The model under review builds one solid part; all positions refer to its coordinate system, in mm. A direction names the side the tool comes from. Coordinates: 2 decimals unless noted, no trailing zeros. Order: outer loops, then holes, each group sorted by start corner. A loop starts at its lowest first (then second) coordinate and runs counter-clockwise, first axis right, second up. Notation, with made-up numbers: (76, 79.5) - (120, 79.5) arc R18 cw to (120, 103.5) - close; hole circle Ø2 at (-24, 71.5). An arc over 180 degrees is marked (long way). Answer in a Markdown table with one row per item.
```python
from build123d import *

# Parameters (mm, degrees)
F0_W     = 17
F0_H     = 17
F1_DEPTH = 1
F2_W     = 14
F2_H     = 14
F3_DEPTH = 1
F4_R     = 0.49999


# Not quite as in the source:
# - a fillet or chamfer is up to 0.001 mm smaller than in the source, because OpenCascade refuses the exact size


with BuildPart() as f1:
    # F0 (on Top) → F1 (new body)
    with BuildSketch(Plane.XY):
        with Locations((-37.4565784931, 18.6608627687)):
            Rectangle(F0_W, F0_H)
    extrude(amount=F1_DEPTH)

    # F2 (on face) → F3 (join)
    with BuildSketch(Plane.XY.offset(1)):
        with Locations((-37.4565784931, 18.6608627687)):
            Rectangle(F2_W, F2_H)
    extrude(amount=F3_DEPTH)

    # F4 (radius 0.5 in the source; OpenCascade refuses exactly that, so slightly less here)
    f4_edges = [f1.edges().sort_by_distance(p)[0] for p in [
        (-37.456578, 25.660863, 2),
        (-44.456578, 18.660863, 2),
        (-44.456578, 18.660863, 1),
        (-37.456578, 25.660863, 1),
        (-37.456578, 11.660863, 2),
        (-37.456578, 10.160863, 1),
        (-45.956578, 18.660863, 1),
        (-45.956578, 18.660863, 0),
        (-45.956578, 27.160863, 0.5),
        (-37.456578, 27.160863, 1),
        (-37.456578, 27.160863, 0),
        (-30.456578, 18.660863, 1),
        (-30.456578, 18.660863, 2),
        (-30.456578, 25.660863, 1.5),
        (-28.956578, 18.660863, 1),
        (-28.956578, 18.660863, 0),
        (-28.956578, 27.160863, 0.5),
        (-28.956578, 10.160863, 0.5),
        (-45.956578, 10.160863, 0.5),
        (-37.456578, 10.160863, 0),
        (-37.456578, 11.660863, 1),
        (-44.456578, 11.660863, 1.5),
        (-30.456578, 11.660863, 1.5),
    ]]
    fillet(f4_edges, radius=F4_R)


solid = f1.part
```
Item 1: We need section C-C, the plane z = 0.75. Write out the cut boundary in (x, y).
Check values:
| item | result |
|---|---|
| outline | (-45.89, 10.66) arc R0.43 ccw to (-45.46, 10.23) - (-29.46, 10.23) arc R0.43 ccw to (-29.02, 10.66) - (-29.02, 26.66) arc R0.43 ccw to (-29.46, 27.09) - (-45.46, 27.09) arc R0.43 ccw to (-45.89, 26.66) - close |
Item 2: To check wall thickness, follow line 1 (Z direction, x = -30, y = 19.5); line 2 (Y direction, x = -33, z = 0.7); line 3 (Y direction, x = -32.5, z = 1.7). State the ranges of each line that lie inside material, in increasing order. Write a range as from..to.
Check values:
| item | result |
|---|---|
| line 1 | 0..1 |
| line 2 | 10.2..27.12 |
| line 3 | 11.7..25.62 |
Item 3: Tool access review of faces 1 (the face through (-38, 11, 1)), 2 (the face through (-38, 19, 2)): name each direction out of +Z, -Z, +X, -X, +Y, -Y from which nothing blocks a thin tool from reaching the whole face with its end or side.
Check values:
| item | result |
|---|---|
| face 1 | +Z |
| face 2 | +Z, +X, -X, +Y, -Y |
